from build123d import *

# Parameters (mm, degrees)
CUT_EXTRUDE1_DEPTH      = 11.344080433
CUT_EXTRUDE1_DEPTH_BACK = 11.344080433
SKETCH2_R               = 0.95
CUT_EXTRUDE2_DEPTH      = 11.344080433
CUT_EXTRUDE2_DEPTH_BACK = 11.344080433


with BuildPart() as part:
    # Sketch1 → Revolve1 (revolve)
    with BuildSketch(Plane.XY):
        Polygon((0, 0), (7, 0), (4, 3), (0, 3), align=None)
    revolve(axis=Axis((0, -1026.355569878, 0), (0, 1, 0)))

    # Sketch2 → Cut-Extrude1 (cut, two sides: drawn at the far end of the back side and taken through both)
    with BuildSketch(Plane(origin=(0, 3, 0), x_dir=(1, 0, 0), z_dir=(0, 1, 0)).offset(-CUT_EXTRUDE1_DEPTH_BACK)):
        with Locations(Location((0, 0, 0), (0, 0, 180))):
            Circle(SKETCH2_R)
    extrude(amount=CUT_EXTRUDE1_DEPTH + CUT_EXTRUDE1_DEPTH_BACK, mode=Mode.SUBTRACT)

    # Sketch3 → Cut-Extrude2 (cut, two sides: drawn at the far end of the back side and taken through both)
    with BuildSketch(Plane(origin=(0, 3, 0), x_dir=(1, 0, 0), z_dir=(0, 1, 0)).offset(-CUT_EXTRUDE2_DEPTH_BACK)):
        with BuildLine():
            Line((-0.8, 0.512347538), (-0.8, 6.95413546))
            ThreePointArc((-0.8, 6.95413546), (0, 7), (0.8, 6.95413546))
            Line((0.8, 6.95413546), (0.8, 0.512347538))
            ThreePointArc((0.8, 0.512347538), (0, 0.95), (-0.8, 0.512347538))
        make_face()
    extrude(amount=CUT_EXTRUDE2_DEPTH + CUT_EXTRUDE2_DEPTH_BACK, mode=Mode.SUBTRACT)


solid = part.part
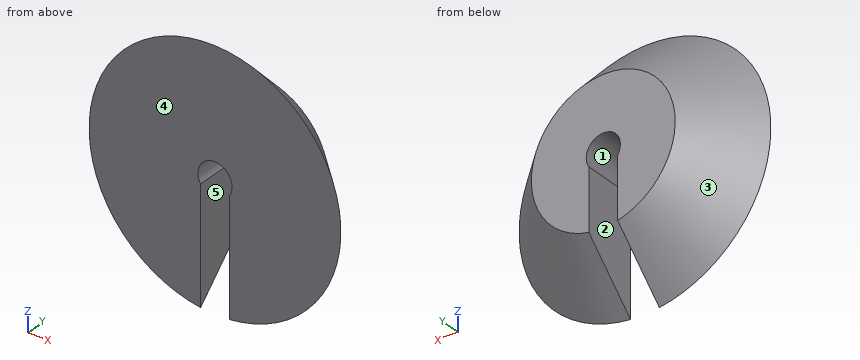
For this review, take the finished solid that the model builds, in its own axes (mm). Face numbers are marked on the shaded views. A direction names the side the tool comes from. Round coordinates to 2 decimals unless told otherwise and drop trailing zeros. Loops run counter-clockwise (first coordinate to the right, second up) from the corner with the lowest first, then second, coordinate; pieces in that order, holes last. Notation, with made-up numbers: (39.5, 37.25) - (68.5, 37.25) arc R25 ccw to (68.5, 57.25) - close; hole circle Ø9 at (-22, -34.5). An arc over 180 degrees is marked (long way). One line per item, written item: value. Start each with the question number.
Item 1: Take a section at C-C (y = 2.2). Give the boundary of the cut face in (x, z).
Item 2: For the marked faces 1 and 2, list the 3-axis set-ups (+Z, -Z, +X, -X, +Y, -Y) from which the entire face can be reached by the end or side of a thin tool; tool diameter is ignored.
Item 3: Take a section at A-A (z = 0). Give the boundary of the cut face in (x, y).
Item 4: Clearance check with flat-ended pins moving along their axes: pin 1 Ø6 at (x, z) = (-0.5, -2) entering from +Y; pin 2 Ø0.9 at (y, z) = (1.5, -2.5) entering from -X; pin 3 Ø1.5 at (y, z) = (2.5, 1.5) entering from -X. State where each tip first meets the part, or that it passes through.
Item 5: The part is to be moulded in two halves that separate along Y. For the marked faces 3, 4 and 5, say which applies: +Y half, -Y half, draft (parallel to the pull), parting line (faces both ways), or undercut.
Item 6: Take a section at B-B (x = 0). Give the boundary of the cut face in (y, z), plus the area to 4 significant figures.
Item 7: For L1, parallel to X at y = 1.4, z = 0; L2, parallel to X at y = 0.9, z = 0; L3, parallel to Y at x = 3.75, z = -1.75, list the stretches that pass through material, from the lowest coordinate up.
Answer below:
1. outline: (-0.8, -4.73) - (-0.8, -0.51) arc R0.95 cw (long way) to (0.8, -0.51) - (0.8, -4.73) arc R4.8 ccw (long way) to start
2. face 1: +Y, -Y
2. face 2: -Z, +Y, -Y
3. outline: (-7, 0) - (-0.95, 0) - (-0.95, 3) - (-4, 3) - close; (0.95, 0) - (7, 0) - (4, 3) - (0.95, 3) - close
4. pin 1: stops at y = 3
4. pin 2: stops at x = -5.44
4. pin 3: stops at x = -5.06
5. face 3: +Y half
5. face 4: -Y half
5. face 5: draft
6. outline: (0, 0.95) - (3, 0.95) - (3, 4) - (0, 7) - close
6. area: 13.65 mm2
7. L1: x = -5.6 to -0.95, 0.95 to 5.6
7. L2: x = -6.1 to -0.95, 0.95 to 6.1
7. L3: y = 0 to 2.86
